from build123d import *

# Parameters (mm, degrees)
BOX016_W        = 430
BOX016_H        = 12
BOX016_DEPTH    = 250
POCKET012_DEPTH = 12
PAD_DEPTH       = 792


with BuildPart() as part:
    # Box016 → Box016 (new body)
    with BuildSketch(Plane(origin=(185, 144, 60), x_dir=(1, 0, 0), z_dir=(0, 0, 1))):
        with Locations((215, 6)):
            Rectangle(BOX016_W, BOX016_H)
    extrude(amount=BOX016_DEPTH)

    # Sketch012 → Pocket012 (cut)
    with BuildSketch(Plane(origin=(185, 144, 60), x_dir=(1, 0, 0), z_dir=(0, -1, 0))):
        Polygon((0, 250), (0, 0), (60, 0), align=None)
        Polygon((430, 250), (430, 0), (370, 0), align=None)
    extrude(amount=-POCKET012_DEPTH, mode=Mode.SUBTRACT)

    # Sketch019 → Pad (new body)
    with BuildSketch(Plane(origin=(185, 156, 60), x_dir=(-1, 0, 0), z_dir=(0, 1, 0))):
        Polygon((-60, 0), (-72, 0), (-12, 250), (0, 250), align=None)
        Polygon((-370, 0), (-430, 250), (-418, 250), (-358, 0), align=None)
    extrude(amount=PAD_DEPTH)


solid = part.part
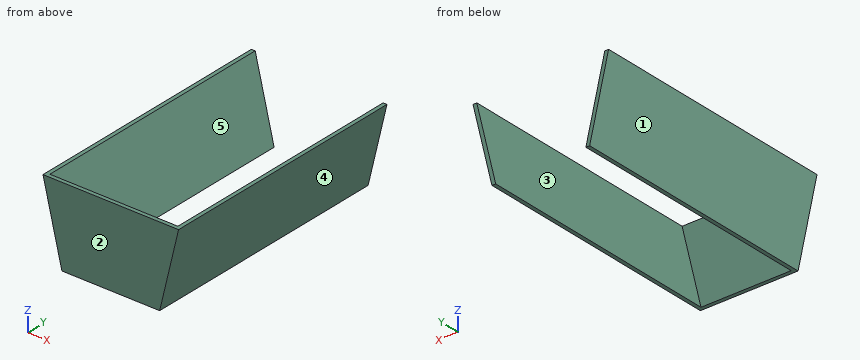
Design review of the part built by this model. Coordinates are the model's own, in mm. Face numbers are marked on the shaded views. A direction names the side the tool comes from. Round coordinates to 2 decimals unless told otherwise and drop trailing zeros. Write each loop counter-clockwise with the first axis right and the second up, starting at its lowest first coordinate (ties: lowest second). Pieces come first, ordered by that corner, then holes. Notation, with made-up numbers: (-22, 83.5) - (19, 83.5) arc R25 cw to (19, 95.5) - close; hole circle Ø11 at (19, 22.25). An arc over 180 degrees is marked (long way). Use a Markdown table: item, result. Add a question column.
1. Mouldability with a two-part tool opening along X and no side actions: class the marked faces 1, 2 and 3 as +X half, -X half, draft (parallel to the pull), parting line (faces both ways), or undercut.
2. Wall thickness on probe 1 along Y at (x, z) = (565.5, 280); probe 2 along X at (y, z) = (292.5, 256); probe 3 along X at (y, z) = (416, 149): over which ranges is each line inside the solid? List them lowest first.
3. For the marked faces 4 and 5, list the 3-axis set-ups (+Z, -Z, +X, -X, +Y, -Y) from which the entire face can be reached by the end or side of a thin tool; tool diameter is ignored.
4. We need section D-D (x = 229.5). State the section outline as (y, z) points, then the cut area to 3 significant figures.
5. We need section A-A (y = 542.5). State the section outline as (x, z) points.
6. Clearance check with flat-ended pins moving along their axes: pin 1 (5 mm diameter, centred on x = 393, z = 201, fed in from +Y); pin 2 (4 mm diameter, centred on y = 563, z = 235, fed in from +X); pin 3 (3 mm diameter, centred on y = 516, z = 89, fed in from +X). State where each tip first meets the part, or that it passes through.
7. We need section B-B (z = 212). State the section outline as (x, y) points.
8. We need section C-C (z = 146). State the section outline as (x, y) points, then the cut area to 3 significant figures.
Output:
| question | item | result |
|---|---|---|
| 1 | face 1 | -X half |
| 1 | face 2 | draft |
| 1 | face 3 | undercut |
| 2 | probe 1 | y = 144 to 156 |
| 2 | probe 2 | x = 197.96 to 209.96, 590.04 to 602.04 |
| 2 | probe 3 | x = 223.64 to 235.64, 564.36 to 576.36 |
| 3 | face 4 | -Z, +X, +Y, -Y |
| 3 | face 5 | +Z, +Y |
| 4 | outline | (144, 124.58) - (948, 124.58) - (948, 174.58) - (156, 174.58) - (156, 310) - (144, 310) - close |
| 4 | area | 41,800 mm2 |
| 5 | outline | (185, 310) - (245, 60) - (257, 60) - (197, 310) - close; (543, 60) - (555, 60) - (615, 310) - (603, 310) - close |
| 6 | pin 1 | stops at y = 156 |
| 6 | pin 2 | stops at x = 597.48 |
| 6 | pin 3 | stops at x = 562.32 |
| 7 | outline | (208.52, 144) - (591.48, 144) - (591.48, 948) - (579.48, 948) - (579.48, 156) - (220.52, 156) - (220.52, 948) - (208.52, 948) - close |
| 8 | outline | (224.36, 144) - (575.64, 144) - (575.64, 948) - (563.64, 948) - (563.64, 156) - (236.36, 156) - (236.36, 948) - (224.36, 948) - close |
| 8 | area | 23,200 mm2 |
